Input: dimensioned drawing with shaded views. Units: mm. Origin: part minimum x, y, z. A direction names the side the tool comes from. Give positions to 0.01 mm unless a question says otherwise; leave off trailing zeros. Order: outer loops, then holes, each group sorted by start corner. A loop starts at its lowest first (then second) coordinate and runs counter-clockwise, first axis right, second up. Notation, with made-up numbers: (-25, 52) - (-9, 52) arc R20 cw to (-9, 88) - close; hole circle Ø3 at (66.5, 0). An arc over 180 degrees is marked (long way). Answer as CSV lines item,"result".
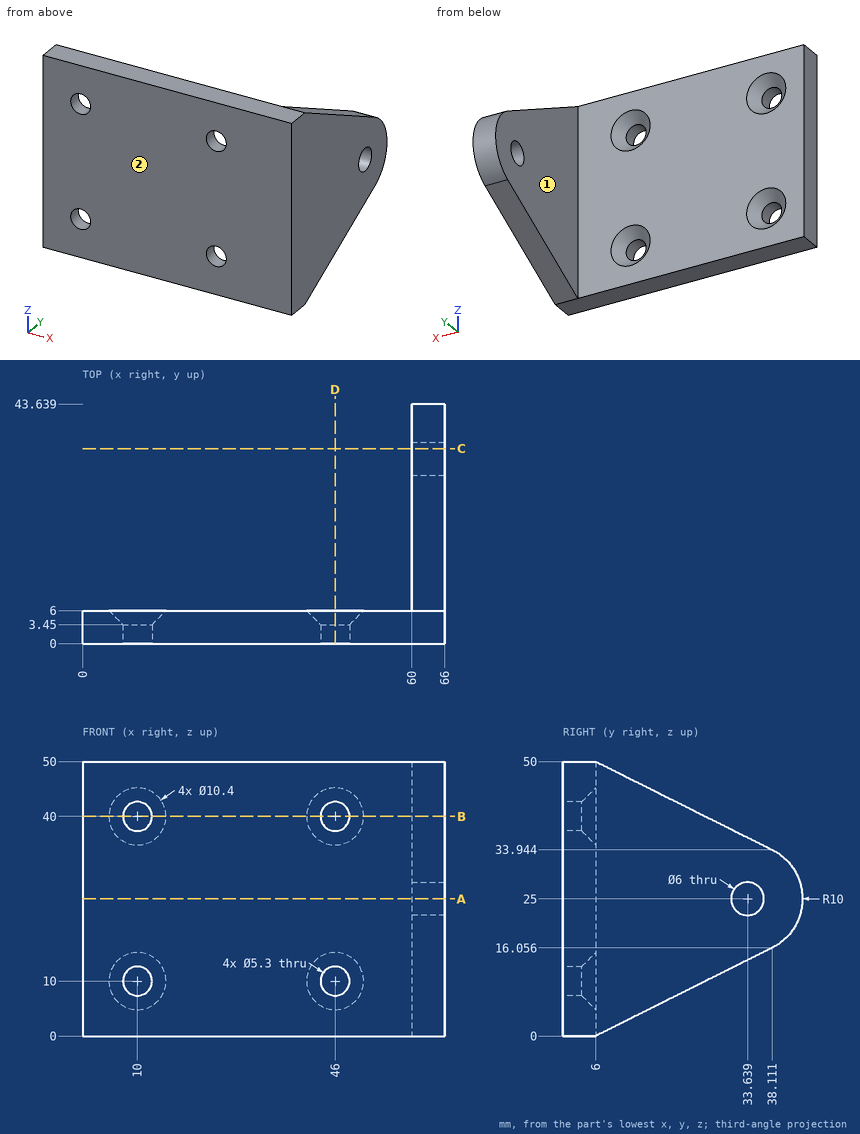
(1) Contact query for flat-ended pins moving along their axis: pin 1 (2 mm diameter, centred on x = 7, z = 23, fed in from +Y); pin 2 (3 mm diameter, centred on x = 46, z = 10, fed in from -Y); pin 3 (8.5 mm diameter, centred on x = 10, z = 40, fed in from +Y). Output: stop coordinate, or through.
Completed:
pin 1,"y = 6"
pin 2,"through"
pin 3,"y = 5.05"
(2) Cut plane C-C (y = 35.5). Return loops of the section in (x, z).
Completed:
outline,"(60, 14.75) - (66, 14.75) - (66, 22.65) - (60, 22.65) - close; (60, 27.35) - (66, 27.35) - (66, 35.25) - (60, 35.25) - close"
(3) Access query for the marked faces 1 and 2. Directions: +Z, -Z, +X, -X, +Y, -Y. A direction counts if a zero-diameter tool reaches every point of the face in a straight line with its end or side. Return the directions, or none.
Completed:
face 1,"+Z, -Z, -X, +Y"
face 2,"+Z, -Z, +X, -X, -Y"
(4) Ray query, line 1 (Z direction, x = 10, y = 2.3); line 2 (Z direction, x = 44.5, y = 4) (1 decimal); line 3 (Y direction, x = 64, z = 25). Return the intervals inside material, ascending. Write a range as from..to.
Completed:
line 1,"0..7.35, 12.65..37.35, 42.65..50"
line 2,"0..7.2, 12.8..37.2, 42.8..50"
line 3,"0..30.64, 36.64..43.64"
(5) Cut plane D-D (x = 46). Return loops of the section in (y, z).
Completed:
outline,"(0, 0) - (6, 0) - (6, 4.8) - (3.45, 7.35) - (0, 7.35) - close; (0, 12.65) - (3.45, 12.65) - (6, 15.2) - (6, 34.8) - (3.45, 37.35) - (0, 37.35) - close; (0, 42.65) - (3.45, 42.65) - (6, 45.2) - (6, 50) - (0, 50) - close"
(6) Cut plane A-A (z = 25). Return loops of the section in (x, y).
Completed:
outline,"(0, 0) - (66, 0) - (66, 30.64) - (60, 30.64) - (60, 6) - (0, 6) - close; (60, 36.64) - (66, 36.64) - (66, 43.64) - (60, 43.64) - close"
(7) Cut plane B-B (z = 40). Return loops of the section in (x, y).
Completed:
outline,"(0, 0) - (7.35, 0) - (7.35, 3.45) - (4.8, 6) - (0, 6) - close; (12.65, 0) - (43.35, 0) - (43.35, 3.45) - (40.8, 6) - (15.2, 6) - (12.65, 3.45) - close; (48.65, 0) - (66, 0) - (66, 26) - (60, 26) - (60, 6) - (51.2, 6) - (48.65, 3.45) - close"
